Read the model definition and answer for the solid it produces. Units are mm, in the model's axes. Give positions to 0.01 mm unless a question says otherwise; leave off trailing zeros. Order: outer loops, then holes, each group sorted by start corner. A loop starts at its lowest first (then second) coordinate and runs counter-clockwise, first axis right, second up. Notation, with made-up numbers: M 55,12 L 97,12 A25 ccw 97,43 Z; hole C -23,48.5 d2. An arc over 180 degrees is marked long. One line per item, written item: value. Start each with the question number.
from build123d import *

# Parameters (mm, degrees)
SKETCH_1_W      = 30
SKETCH_1_H      = 19
SKETCH_1_R      = 1.5
EXTRUDE_1_DEPTH = 1.5
CHAMFER_1_SIZE  = 2


with BuildPart() as part:
    # Эскиз1 → Бобышка-Вытянуть1 (new body)
    with BuildSketch(Plane(origin=(0, 0, 0), x_dir=(1, 0, 0), z_dir=(0, 1, 0))):
        Rectangle(SKETCH_1_W, SKETCH_1_H)
        with Locations(Location((11.9, 6.75, 0), (0, 0, 270))):
            Circle(SKETCH_1_R, mode=Mode.SUBTRACT)
        with Locations(Location((11.9, -6.75, 0), (0, 0, 270))):
            Circle(SKETCH_1_R, mode=Mode.SUBTRACT)
    extrude(amount=EXTRUDE_1_DEPTH)

    # Фаска1
    chamfer_1_edges = [part.edges().sort_by_distance(p)[0] for p in [
        (-15, 0.75, -9.5),
        (15, 0.75, -9.5),
        (15, 0.75, 9.5),
        (-15, 0.75, 9.5),
    ]]
    chamfer(chamfer_1_edges, length=CHAMFER_1_SIZE)


solid = part.part
Q1. Find section D-D, the plane z = 6.25. Give the vertices of the cut face in (x, y), then the cut area to 3 significant figures.
Q2. Find section C-C, the plane y = 1.05. Give the vertices of the cut face in (x, z).
Q3. Determine the mould class of faces 1 (the flat face through (0, 1, 9.5)), 2 (the cylindrical face through (11.97, 0.74, -8.25)), 3 (the flat face through (15, 1, 0)) for opening direction X: released by +X, released by -X, zero draft, split by the parting line, or undercut.
Q4. Consider probe 1 along X at (y, z) = (0.6, -6.75); probe 2 along X at (y, z) = (0.55, -5.5); probe 3 along X at (y, z) = (0.5, -8.5). Determine where each line is inside the solid, lowest interval first.
Q5. Find section A-A, the plane z = -6.75. Give the vertices of the cut face in (x, y).
Q6. Find section B-B, the plane x = 11.9. Give the vertices of the cut face in (y, z).
Q7. This flat-tipped pin is pushed along its axis until it touches: pin 1 (1.8 mm diameter, centred on x = 11.9, z = 6.75, fed in from -Y). Where does it stop, or does it pass through?
Evaluation:
1. outline: M -15,0 L 10.49,0 L 10.49,1.5 L -15,1.5 Z; M 13.31,0 L 15,0 L 15,1.5 L 13.31,1.5 Z
1. area: 40.8 mm2
2. outline: M -15,-7.5 L -13,-9.5 L 13,-9.5 L 15,-7.5 L 15,7.5 L 13,9.5 L -13,9.5 L -15,7.5 Z; hole C 11.9,-6.75 d3; hole C 11.9,6.75 d3
3. face 1: zero draft
3. face 2: undercut
3. face 3: released by +X
4. probe 1: -15 to 10.4, 13.4 to 15
4. probe 2: -15 to 11.07, 12.73 to 15
4. probe 3: -14 to 14
5. outline: M -15,0 L 10.4,0 L 10.4,1.5 L -15,1.5 Z; M 13.4,0 L 15,0 L 15,1.5 L 13.4,1.5 Z
6. outline: M 0,-9.5 L 1.5,-9.5 L 1.5,-8.25 L 0,-8.25 Z; M 0,-5.25 L 1.5,-5.25 L 1.5,5.25 L 0,5.25 Z; M 0,8.25 L 1.5,8.25 L 1.5,9.5 L 0,9.5 Z
7. pin 1: through
